Verification items for the finished model (mm, model axes). Coordinates: 2 decimals unless noted, no trailing zeros. Order: outer loops, then holes, each group sorted by start corner. A loop starts at its lowest first (then second) coordinate and runs counter-clockwise, first axis right, second up. Notation, with made-up numbers: M 41,85 L 55,85 A24 ccw 55,105 Z; hole C 85.25,73 d2. An arc over 180 degrees is marked long. Answer as a JSON object with one key per item and string values. Group by question number.
(1) Cross-section at C-C (y = -0.95). Enter the section's corners in (x, z), plus the area to 3 significant figures.
(2) Material ranges on line 1 (Y direction, x = 17.5, z = 8.25); line 2 (X direction, y = -0.9, z = -6.5); line 3 (Z direction, x = -4, y = 0.3), recorded low to high.
(3) Cross-section at A-A (z = -6.5). Enter the section's corners in (x, y).
(4) Cross-section at B-B (x = -0.5). Enter the section's corners in (y, z), plus the area to 3 significant figures.
(5) Cross-section at D-D (z = 6). Enter the section's corners in (x, y), plus the area to 3 significant figures.
(6) Gauge pin test, flat ends, axial feed: pin 1 Ø2.5 at (x, z) = (19.52, 7.66) entering from -Y; pin 2 Ø0.8 at (x, y) = (20.5, -0.5) entering from +Z; pin 3 Ø0.5 at (y, z) = (-1, 5) entering from +X. Record the tip position at first contact, or that the pin passes through.
from build123d import *

# Parameters (mm, degrees)
EXTRUDE_1_DEPTH     = 0.5
EXTRUDE_2_DEPTH     = 0.5
SKETCH_3_W          = 32.2
SKETCH_3_H          = 15.4
EXTRUDE_3_DEPTH     = 0.5
EXTRUDE_4_DEPTH     = 1.8
SKETCH_7_R          = 1.15
CUT_EXTRUDE_1_DEPTH = 10


with BuildPart() as part:
    # Эскиз1 → Бобышка-Вытянуть1 (new body)
    with BuildSketch(Plane(origin=(0, 0, 0), x_dir=(1, 0, 0), z_dir=(0, 1, 0))):
        with BuildLine():
            Line((22.815864902, 9.839807024), (-22.784135098, 9.839807024))
            Line((-22.784135098, 9.839807024), (-23.684135098, 8.939807024))
            Line((-23.684135098, 8.939807024), (-23.684135098, -8.260192976))
            Line((-23.684135098, -8.260192976), (-22.784135098, -9.160192976))
            Line((-22.784135098, -9.160192976), (21.215864902, -9.160192976))
            Line((21.215864902, -9.160192976), (23.315864902, -7.060192976))
            Line((23.315864902, -7.060192976), (23.315864902, -3.260192976))
            Line((23.315864902, -3.260192976), (23.029007645, -3.260192976))
            ThreePointArc((23.029007645, -3.260192976), (22.159773793, -4.027024735), (21.188848248, -4.660192976))
            Line((21.188848248, -4.660192976), (21.188848248, -5.660192976))
            Line((21.188848248, -5.660192976), (19.888848248, -5.660192976))
            Line((19.888848248, -5.660192976), (19.888848248, -4.660192976))
            Line((19.888848248, -4.660192976), (17.315864902, -4.660192976))
            Line((17.315864902, -4.660192976), (17.315864902, -8.360192976))
            Line((17.315864902, -8.360192976), (-18.884135098, -8.360192976))
            Line((-18.884135098, -8.360192976), (-18.884135098, -6.660192976))
            Line((-18.884135098, -6.660192976), (-19.684135098, -5.860192976))
            Line((-19.684135098, -5.860192976), (-19.684135098, 6.539807024))
            Line((-19.684135098, 6.539807024), (-18.884135098, 7.339807024))
            Line((-18.884135098, 7.339807024), (-18.884135098, 9.039807024))
            Line((-18.884135098, 9.039807024), (17.315864902, 9.039807024))
            Line((17.315864902, 9.039807024), (17.315864902, 8.539807024))
            ThreePointArc((17.315864902, 8.539807024), (18.329503431, 8.456385882), (19.315864902, 8.208367324))
            Line((19.315864902, 8.208367324), (19.315864902, 9.139807024))
            Line((19.315864902, 9.139807024), (21.530126403, 9.139807024))
            ThreePointArc((21.530126403, 9.139807024), (22.315698775, 8.584938027), (23.029007645, 7.939807024))
            Line((23.029007645, 7.939807024), (23.315864902, 7.939807024))
            Line((23.315864902, 7.939807024), (23.315864902, 9.339807024))
            Line((23.315864902, 9.339807024), (22.815864902, 9.839807024))
        make_face()
        with BuildLine():
            ThreePointArc((18.565864902, -7.660192976), (19.515864902, -8.610192976), (20.465864902, -7.660192976))
            ThreePointArc((20.465864902, -7.660192976), (19.515864902, -6.710192976), (18.565864902, -7.660192976))
        make_face(mode=Mode.SUBTRACT)
        with BuildLine():
            ThreePointArc((-22.034135098, -7.660192976), (-21.084135098, -8.610192976), (-20.134135098, -7.660192976))
            ThreePointArc((-20.134135098, -7.660192976), (-21.084135098, -6.710192976), (-22.034135098, -7.660192976))
        make_face(mode=Mode.SUBTRACT)
        with BuildLine():
            ThreePointArc((-22.034135098, 8.339807024), (-21.084135098, 7.389807024), (-20.134135098, 8.339807024))
            ThreePointArc((-20.134135098, 8.339807024), (-21.084135098, 9.289807024), (-22.034135098, 8.339807024))
        make_face(mode=Mode.SUBTRACT)
    extrude(amount=EXTRUDE_1_DEPTH)

    # Эскиз2 → Бобышка-Вытянуть2 (add)
    with BuildSketch(Plane(origin=(0, 0, 0), x_dir=(-1, 0, 0), z_dir=(0, -1, 0))):
        Polygon((-17.315864902, -4.660192976), (-17.315864902, 9.839807024), (-22.815864902, 9.839807024), (-23.315864902, 9.339807024), (-23.315864902, -7.060192976), (-21.188848248, -5.660192976), (-17.315864902, -5.660192976), align=None)
    extrude(amount=-EXTRUDE_2_DEPTH)

    # Эскиз3 → Бобышка-Вытянуть3 (add)
    with BuildSketch(Plane(origin=(0, 0, 0), x_dir=(-1, 0, 0), z_dir=(0, -1, 0))):
        Polygon((18.884135098, -8.360192976), (18.884135098, -7.760192976), (19.728041262, -7.760192976), (19.728041262, 8.039807024), (18.884135098, 8.039807024), (18.884135098, 9.039807024), (-17.315864902, 9.039807024), (-17.315864902, -8.360192976), align=None)
        with Locations((2.384135098, 0.339807024)):
            Rectangle(SKETCH_3_W, SKETCH_3_H, mode=Mode.SUBTRACT)
    extrude(amount=-EXTRUDE_3_DEPTH)

    # Эскиз6 → Бобышка-Вытянуть4 (add)
    with BuildSketch(Plane(origin=(0, 0, 0), x_dir=(1, 0, 0), z_dir=(0, 1, 0))):
        Polygon((23.315864902, 7.821832851), (23.315864902, -3.062056468), (22.999687869, -3.062056468), (21.261580991, -4.424599137), (21.024758243, -4.424599137), (21.024758243, -5.416287347), (20.030773613, -5.416287347), (20.030773613, -4.424599137), (19.718020582, -4.424599137), (19.718020582, 8.99333189), (21.530126403, 8.99333189), (22.952461546, 7.821832851), align=None)
    extrude(amount=-EXTRUDE_4_DEPTH)

    # Эскиз7 → Вырез-Вытянуть1 (cut)
    with BuildSketch(Plane(origin=(0, 0.5, 0), x_dir=(1, 0, 0), z_dir=(0, 1, 0))):
        with Locations(Location((-21.084135098, 8.339807024, 0), (0, 0, 270))):
            Circle(SKETCH_7_R)
        with Locations(Location((-21.084135098, -7.660192976, 0), (0, 0, 270))):
            Circle(SKETCH_7_R)
        with Locations(Location((19.515864902, -7.660192976, 0), (0, 0, 270))):
            Circle(SKETCH_7_R)
    extrude(amount=-CUT_EXTRUDE_1_DEPTH, mode=Mode.SUBTRACT)


solid = part.part
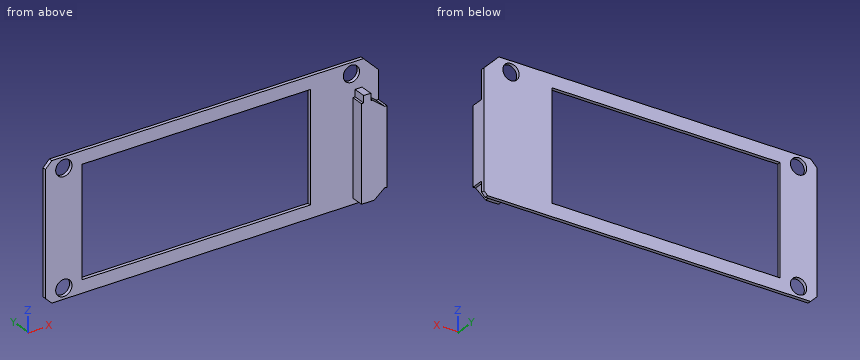
Taken from the geometry:
{
 "1": {"outline": "M 19.72,-8.99 L 21.53,-8.99 L 22.95,-7.82 L 23.32,-7.82 L 23.32,3.06 L 23,3.06 L 21.26,4.42 L 21.02,4.42 L 21.02,5.42 L 20.03,5.42 L 20.03,4.42 L 19.72,4.42 Z", "area": "46.4 mm²"},
 "2": {"line 1": "y = 0 to 0.5", "line 2": "x = 19.72 to 23.32", "line 3": "z = -9.84 to -8.04, 7.36 to 9.16"},
 "3": {"outline": "M -23.68,0 L -18.48,0 L -18.48,0.5 L -23.68,0.5 Z; M 13.72,0 L 19.72,0 L 19.72,-1.8 L 23.32,-1.8 L 23.32,0.5 L 13.72,0.5 Z"},
 "4": {"outline": "M 0,-9.84 L 0.5,-9.84 L 0.5,-8.04 L 0,-8.04 Z; M 0,7.36 L 0.5,7.36 L 0.5,9.16 L 0,9.16 Z", "area": "1.80 mm²"},
 "5": {"outline": "M -23.68,0 L -18.48,0 L -18.48,0.5 L -23.68,0.5 Z; M 13.72,0 L 23.32,0 L 23.32,0.5 L 13.72,0.5 Z", "area": "7.40 mm²"},
 "6": {"pin 1": "stops at y = 0", "pin 2": "stops at z = 5.42", "pin 3": "stops at x = 21.02"}
}
